Part print with two shaded views. Sizes in mm from the minimum x, y, z corner. A direction names the side the tool comes from. Round coordinates to 2 decimals unless told otherwise and drop trailing zeros. Loops run counter-clockwise (first coordinate to the right, second up) from the corner with the lowest first, then second, coordinate; pieces in that order, holes last.
(1) Tool access for the marked faces 5, 6 and 7: list every direction of +Z, -Z, +X, -X, +Y, -Y with a clear straight run to the whole face (end or side of a thin tool).
(2) Probe probe 1 along Y at (x, z) = (21, 13); probe 2 along Z at (x, y) = (6, 10); probe 3 along X at (y, z) = (5, 4). List the from-to ranges inside material, lowest first.
(3) Flat gauge pins, fed straight in: pin 1 (8 mm diameter, centred on x = 37, y = 21, fed in from -Z); pin 2 (3.5 mm diameter, centred on x = 37, y = 21, fed in from -Z); pin 3 (1 mm diameter, centred on y = 25, z = 4.5, fed in from -X); pin 4 (4 mm diameter, centred on x = 5.5, y = 21, fed in from -Z). Where does each tip first touch, or does it go through?
(4) Mould opens along X. For the marked faces 1, 2, 3 and 4 say: +X half, -X half, draft (parallel to the pull), parting line (faces both ways), or undercut.
(5) Cut at C-C on z = 10.5. List the corners of the cut face in (x, y).
(6) Cut at A-A on x = 21. Count the separate pieces of the cut face and the enclosed holes in it, then the cut area to 3 significant figures.
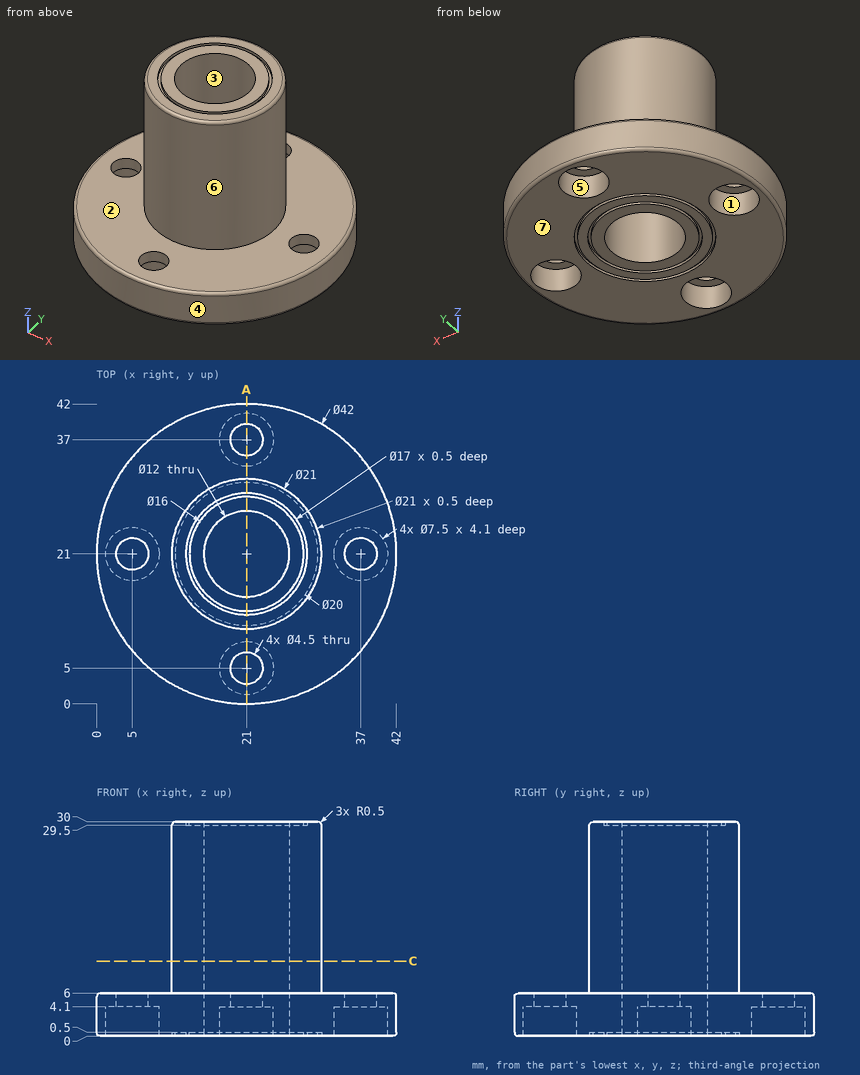
Final values:
1. face 5: -Z
1. face 6: +Z
1. face 7: -Z, +X, -X, +Y, -Y
2. probe 1: y = 10.5 to 15, 27 to 31.5
2. probe 2: z = 0 to 6
2. probe 3: x = 7.4 to 17.25, 24.75 to 34.6
3. pin 1: stops at z = 0
3. pin 2: passes through
3. pin 3: stops at x = 0.29
3. pin 4: stops at z = 4.1
4. face 1: undercut
4. face 2: draft
4. face 3: undercut
4. face 4: parting line
5. outline: circle Ø21 at (21, 21); hole circle Ø12 at (21, 21)
6. separate pieces: 4
6. enclosed holes: 0
6. area: 316 mm2
